from build123d import *

# Parameters (mm, degrees)
SKETCH1_W           = 66.4
SKETCH1_H           = 5.8
BOSS_EXTRUDE1_DEPTH = 25
SKETCH3_R           = 5.28
SKETCH3_W           = 11.88
SKETCH3_H           = 6.07
CUT_EXTRUDE3_DEPTH  = 6.8


with BuildPart() as part:
    # Sketch1 → Boss-Extrude1 (new body)
    with BuildSketch(Plane.XY):
        with Locations((0, -59.6)):
            Rectangle(SKETCH1_W, SKETCH1_H)
    extrude(amount=BOSS_EXTRUDE1_DEPTH)

    # Sketch3 → Cut-Extrude3 (cut, through all)
    with BuildSketch(Plane(origin=(0, -56.7, 0), x_dir=(1, 0, 0), z_dir=(0, 1, 0))):
        with Locations((-23.26, -15.500000019)):
            Circle(SKETCH3_R)
        with Locations((23.26, -15.500000019)):
            Rectangle(SKETCH3_W, SKETCH3_H)
    extrude(amount=-CUT_EXTRUDE3_DEPTH, mode=Mode.SUBTRACT)


solid = part.part
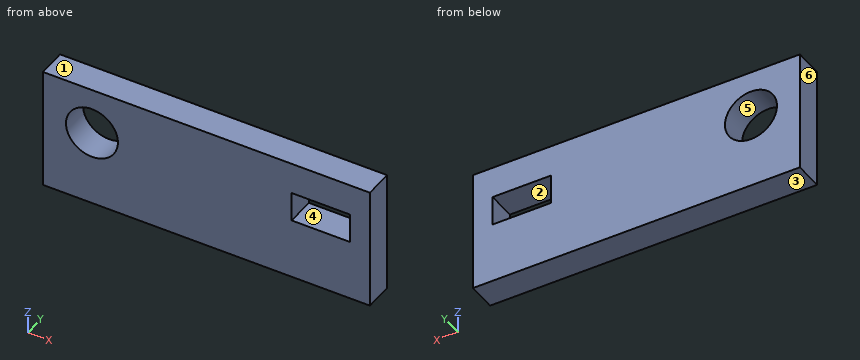
Could you check a few things on this model? Use its own coordinates, in mm. Face numbers are marked on the shaded views. A direction names the side the tool comes from. Coordinates: 2 decimals unless noted, no trailing zeros. Order: outer loops, then holes, each group sorted by start corner. A loop starts at its lowest first (then second) coordinate and runs counter-clockwise, first axis right, second up. Notation, with made-up numbers: (23.25, 58) -> (51.25, 58) arc R34 ccw to (51.25, 92) -> close; hole circle Ø9 at (70.5, 75). An arc over 180 degrees is marked (long way). One line per question, with ' | ' between items.
Q1. Imagine slicing it at A-A on z = 15.5. Please give me the cut outline in (x, y).
Return value:
outline: (-33.2, -62.5) -> (-28.54, -62.5) -> (-28.54, -56.7) -> (-33.2, -56.7) -> close; (-17.98, -62.5) -> (17.32, -62.5) -> (17.32, -56.7) -> (-17.98, -56.7) -> close; (29.2, -62.5) -> (33.2, -62.5) -> (33.2, -56.7) -> (29.2, -56.7) -> close
Q2. If I drill on L1, parallel to Z at x = -23.26, y = -58.9; L2, parallel to Z at x = 19, y = -60.35 (3 decimals), over which ranges is the centre line in solid material (lowest first)?
Return value:
L1: 0 to 10.22, 20.78 to 25 | L2: 0 to 12.465, 18.535 to 25
Q3. Thinking about a two-plate mould opening in X: for the marked faces 3, 4, 5 and 6, which applies, pulls with the +X half, pulls with the -X half, needs draft (parallel to the pull), parting line crosses it, or undercut?
Return value:
face 3: needs draft | face 4: undercut | face 5: undercut | face 6: pulls with the -X half
Q4. Imagine slicing it at C-C on y = -59.9. Please give me the cut outline in (x, z) (3 decimals).
Return value:
outline: (-33.2, 0) -> (33.2, 0) -> (33.2, 25) -> (-33.2, 25) -> close; hole circle Ø10.56 at (-23.26, 15.5); hole (17.32, 12.465) -> (29.2, 12.465) -> (29.2, 18.535) -> (17.32, 18.535) -> close
Q5. On a 3-axis mill with a long thin cutter (end or side, diameter ignored), from which of +Z, -Z, +X, -X, +Y, -Y can I reach the whole of each face in a straight line? I mean the marked faces 1 and 2. Say none if no direction works.
Return value:
face 1: +Z, +X, -X, +Y, -Y | face 2: +Y, -Y
Q6. Imagine slicing it at D-D on z = 19.5. Please give me the cut outline in (x, y).
Return value:
outline: (-33.2, -62.5) -> (-26.71, -62.5) -> (-26.71, -56.7) -> (-33.2, -56.7) -> close; (-19.81, -62.5) -> (33.2, -62.5) -> (33.2, -56.7) -> (-19.81, -56.7) -> close
Q7. Imagine slicing it at B-B on x = -23.26. Please give me the cut outline in (y, z), and give its area (3 significant figures).
Return value:
outline: (-62.5, 0) -> (-56.7, 0) -> (-56.7, 10.22) -> (-62.5, 10.22) -> close; (-62.5, 20.78) -> (-56.7, 20.78) -> (-56.7, 25) -> (-62.5, 25) -> close | area: 83.8 mm²
